```python
from build123d import *

# Parameters (mm, degrees)
BOSS_EXTRUDE1_DEPTH = 28.5
CUT_EXTRUDE1_DEPTH  = 26.5
CUT_EXTRUDE2_DEPTH  = 8
CUT_EXTRUDE3_DEPTH  = 3


with BuildPart() as part:
    # Sketch1 → Boss-Extrude1 (new body)
    with BuildSketch(Plane(origin=(0, 0, 0), x_dir=(1, 0, 0), z_dir=(0, 1, 0))):
        with BuildLine():
            Line((-35, 76.508623254), (-35, 3.969028671))
            ThreePointArc((-35, 3.969028671), (-34.63575277, 2.989199275), (-33.719912473, 2.485236737))
            ThreePointArc((-33.719912473, 2.485236737), (0, 0), (33.719912473, 2.485236737))
            ThreePointArc((33.719912473, 2.485236737), (34.63575277, 2.989199275), (35, 3.969028671))
            Line((35, 3.969028671), (35, 76.508623254))
            ThreePointArc((35, 76.508623254), (34.96885474, 76.812705074), (34.876712329, 77.104159284))
            ThreePointArc((34.876712329, 77.104159284), (32, 91), (34.876712329, 104.895840716))
            ThreePointArc((34.876712329, 104.895840716), (34.96885474, 105.187294926), (35, 105.491376746))
            Line((35, 105.491376746), (35, 169.530971329))
            ThreePointArc((35, 169.530971329), (34.63575277, 170.510800725), (33.719912473, 171.014763263))
            ThreePointArc((33.719912473, 171.014763263), (0, 173.5), (-33.719912473, 171.014763263))
            ThreePointArc((-33.719912473, 171.014763263), (-34.63575277, 170.510800725), (-35, 169.530971329))
            Line((-35, 169.530971329), (-35, 105.491376746))
            ThreePointArc((-35, 105.491376746), (-34.96885474, 105.187294926), (-34.876712329, 104.895840716))
            ThreePointArc((-34.876712329, 104.895840716), (-32, 91), (-34.876712329, 77.104159284))
            ThreePointArc((-34.876712329, 77.104159284), (-34.96885474, 76.812705074), (-35, 76.508623254))
        make_face()
    extrude(amount=BOSS_EXTRUDE1_DEPTH)

    # Sketch2 → Cut-Extrude1 (cut)
    with BuildSketch(Plane(origin=(0, 0, 0), x_dir=(1, 0, 0), z_dir=(0, 1, 0))):
        with BuildLine():
            Line((20, 55.5), (20, 106.320508076))
            ThreePointArc((20, 106.320508076), (19.659258263, 108.908698527), (18.660254038, 111.320508076))
            Line((18.660254038, 111.320508076), (13.339745962, 120.535898385))
            ThreePointArc((13.339745962, 120.535898385), (12.340741737, 122.947707934), (12, 125.535898385))
            Line((12, 125.535898385), (12, 147))
            ThreePointArc((12, 147), (0, 159), (-12, 147))
            Line((-12, 147), (-12, 125.535898385))
            ThreePointArc((-12, 125.535898385), (-12.340741737, 122.947707934), (-13.339745962, 120.535898385))
            Line((-13.339745962, 120.535898385), (-18.660254038, 111.320508076))
            ThreePointArc((-18.660254038, 111.320508076), (-19.659258263, 108.908698527), (-20, 106.320508076))
            Line((-20, 106.320508076), (-20, 55.5))
            ThreePointArc((-20, 55.5), (-20.194193243, 53.538838649), (-20.769230769, 51.653846154))
            ThreePointArc((-20.769230769, 51.653846154), (0, 20.5), (20.769230769, 51.653846154))
            ThreePointArc((20.769230769, 51.653846154), (20.194193243, 53.538838649), (20, 55.5))
        make_face()
    extrude(amount=CUT_EXTRUDE1_DEPTH, mode=Mode.SUBTRACT)

    # Sketch3 → Cut-Extrude2 (cut)
    with BuildSketch(Plane(origin=(0, 0, 0), x_dir=(1, 0, 0), z_dir=(0, 1, 0))):
        with BuildLine():
            ThreePointArc((-7.988063039, 156.239224138), (0, 120), (7.988063039, 156.239224138))
            ThreePointArc((7.988063039, 156.239224138), (7.304821226, 156.588253024), (6.650349133, 156.988636364))
            ThreePointArc((6.650349133, 156.988636364), (0, 159), (-6.650349133, 156.988636364))
            ThreePointArc((-6.650349133, 156.988636364), (-7.304821226, 156.588253024), (-7.988063039, 156.239224138))
        make_face()
    extrude(amount=CUT_EXTRUDE2_DEPTH, mode=Mode.SUBTRACT)

    # Sketch4 → Cut-Extrude3 (cut)
    with BuildSketch(Plane(origin=(0, 0, 0), x_dir=(1, 0, 0), z_dir=(0, 1, 0))):
        with BuildLine():
            Line((25, 51.426149773), (25, 130.573850227))
            ThreePointArc((25, 130.573850227), (25.06968726, 131.752361529), (25.277777778, 132.914447386))
            ThreePointArc((25.277777778, 132.914447386), (0, 165), (-25.277777778, 132.914447386))
            ThreePointArc((-25.277777778, 132.914447386), (-25.06968726, 131.752361529), (-25, 130.573850227))
            Line((-25, 130.573850227), (-25, 51.426149773))
            ThreePointArc((-25, 51.426149773), (-25.06968726, 50.247638471), (-25.277777778, 49.085552614))
            ThreePointArc((-25.277777778, 49.085552614), (0, 17), (25.277777778, 49.085552614))
            ThreePointArc((25.277777778, 49.085552614), (25.06968726, 50.247638471), (25, 51.426149773))
        make_face()
    extrude(amount=CUT_EXTRUDE3_DEPTH, mode=Mode.SUBTRACT)

    # Sketch5 → Cut-Revolve1 (revolve, cut)
    with BuildSketch(Plane(origin=(0, 0, 0), x_dir=(0, 0, -1), z_dir=(1, 0, 0))):
        Polygon((6, 28.5), (11, 28.5), (11, 22.5), (8.75, 22.5), (8.75, 0), (6, 0), align=None)
    revolve(axis=Axis((0, 0, -6), (0, 1, 0)), mode=Mode.SUBTRACT)

    # Sketch6 → Cut-Revolve2 (revolve, cut)
    with BuildSketch(Plane(origin=(29, 0, 0), x_dir=(0, 0, -1), z_dir=(1, 0, 0))):
        Polygon((106.5, 28.5), (111.5, 28.5), (111.5, 22.5), (109.25, 22.5), (109.25, 0), (106.5, 0), align=None)
    revolve(axis=Axis((29, 0, -106.5), (0, 1, 0)), mode=Mode.SUBTRACT)

    # Sketch7 → Cut-Revolve3 (revolve, cut)
    with BuildSketch(Plane(origin=(29, 0, 0), x_dir=(0, 0, -1), z_dir=(1, 0, 0))):
        Polygon((149, 28.5), (154, 28.5), (154, 22.5), (151.75, 22.5), (151.75, 0), (149, 0), align=None)
    revolve(axis=Axis((29, 0, -149), (0, 1, 0)), mode=Mode.SUBTRACT)

    # Sketch8 → Cut-Revolve4 (revolve, cut)
    with BuildSketch(Plane(origin=(-29, 0, 0), x_dir=(0, 0, -1), z_dir=(1, 0, 0))):
        Polygon((106.5, 28.5), (111.5, 28.5), (111.5, 22.5), (109.25, 22.5), (109.25, 0), (106.5, 0), align=None)
    revolve(axis=Axis((-29, 0, -106.5), (0, 1, 0)), mode=Mode.SUBTRACT)

    # Sketch9 → Cut-Revolve5 (revolve, cut)
    with BuildSketch(Plane(origin=(-29, 0, 0), x_dir=(0, 0, -1), z_dir=(1, 0, 0))):
        Polygon((149, 28.5), (154, 28.5), (154, 22.5), (151.75, 22.5), (151.75, 0), (149, 0), align=None)
    revolve(axis=Axis((-29, 0, -149), (0, 1, 0)), mode=Mode.SUBTRACT)

    # Sketch10 → Cut-Revolve6 (revolve, cut)
    with BuildSketch(Plane.XY.offset(-158)):
        Polygon((19, 28.5), (22, 28.5), (21.4585, 27.9585), (21.4585, 12), (19, 10.580584363), align=None)
    revolve(axis=Axis((19, 10.580584363, -158), (0, 1, 0)), mode=Mode.SUBTRACT)

    # Sketch11 → Cut-Revolve7 (revolve, cut)
    with BuildSketch(Plane.XY.offset(-158)):
        Polygon((-19, 28.5), (-16, 28.5), (-16.5415, 27.9585), (-16.5415, 12), (-19, 10.580584363), align=None)
    revolve(axis=Axis((-19, 10.580584363, -158), (0, 1, 0)), mode=Mode.SUBTRACT)

    # Sketch12 → Cut-Revolve8 (revolve, cut)
    with BuildSketch(Plane.XY.offset(-120)):
        Polygon((19, 28.5), (22, 28.5), (21.4585, 27.9585), (21.4585, 12), (19, 10.580584363), align=None)
    revolve(axis=Axis((19, 10.580584363, -120), (0, 1, 0)), mode=Mode.SUBTRACT)

    # Sketch13 → Cut-Revolve9 (revolve, cut)
    with BuildSketch(Plane.XY.offset(-120)):
        Polygon((-19, 28.5), (-16, 28.5), (-16.5415, 27.9585), (-16.5415, 12), (-19, 10.580584363), align=None)
    revolve(axis=Axis((-19, 10.580584363, -120), (0, 1, 0)), mode=Mode.SUBTRACT)


solid = part.part
```
The model under review builds one solid part; all positions refer to its coordinate system, in mm. A direction names the side the tool comes from. Round coordinates to 2 decimals unless told otherwise and drop trailing zeros. Loops run counter-clockwise (first coordinate to the right, second up) from the corner with the lowest first, then second, coordinate; pieces in that order, holes last.
1) Tool access review of faces 4 (the face through (16.04, 14.59, -115.86)), 5 (the face through (18.47, 19.87, -117.6)), 6 (the face through (1.05, 11.09, -8.54)): name each direction out of +Z, -Z, +X, -X, +Y, -Y from which nothing blocks a thin tool from reaching the whole face with its end or side.
Values follow:
face 4: -Y
face 5: +Y
face 6: +Y, -Y
2) Consider section A-A on z = -43. State the section outline as (x, y) points.
Values follow:
outline: (-35, 0) - (-26, 0) - (-26, 3) - (-22.5, 3) - (-22.5, 26.5) - (22.5, 26.5) - (22.5, 3) - (26, 3) - (26, 0) - (35, 0) - (35, 28.5) - (-35, 28.5) - close
3) Clearance check with flat-ended pins moving along their axes: P1, Ø6, axis at x = 29, z = -106.5, coming from the +Y side; P2, Ø4, axis at x = 19, z = -158, coming from the +Y side; P3, Ø6, axis at x = -10.5, z = -145.5, coming from the -Y side. State where each tip first meets the part, or that it passes through.
Values follow:
P1: stops at y = 22.5
P2: stops at y = 11.74
P3: stops at y = 8
4) The part is to be moulded in two halves that separate along Z. For faces 1 (the face through (-35, 14, -138)), 2 (the face through (0, 14, 0)), 3 (the face through (32, 14, -91)), say which applies: pulls with the +Z half, pulls with the -Z half, needs draft (parallel to the pull), parting line crosses it, or undercut.
Values follow:
face 1: needs draft
face 2: pulls with the +Z half
face 3: undercut
5) Wall thickness on line 1 along X through (y, z) = (10.75, -6); line 2 along X through (y, z) = (10, -56.5); line 3 along Z through (x, y) = (29, 24.5): over which ranges is each line inside the solid? List them lowest first.
Values follow:
line 1: x = -35 to -2.75, 2.75 to 35
line 2: x = -35 to -20, 20 to 35
line 3: z = -171.66 to -154, -144 to -111.5, -101.5 to -1.84
6) Consider section B-B on y = 20.5. Give the number of separate pieces and of enclosed holes in the cut face, then the cut area to 3 significant figures.
Values follow:
separate pieces: 1
enclosed holes: 10
area: 6,990 mm2
7) Consider section C-C on z = -139. State the section outline as (x, y) points.
Values follow:
outline: (-35, 0) - (-26, 0) - (-26, 3) - (-19, 3) - (-19, 8) - (-12, 8) - (-12, 26.5) - (12, 26.5) - (12, 8) - (19, 8) - (19, 3) - (26, 3) - (26, 0) - (35, 0) - (35, 28.5) - (-35, 28.5) - close
